from build123d import *

# Parameters (mm, degrees)
SKETCH1_R                     = 22.5
PLATE_DEPTH                   = 5
OPENING_START                 = 1.5
OPENING_FOR_SCREW_DEPTH       = 5
SKETCH7_R                     = 1.75
SCREW_HOLE_DEPTH              = 5
CIRPATTERN20_COUNT            = 3
SKETCH10_W                    = 45
SKETCH10_H                    = 1
SKETCH10_W_2                  = 1
SKETCH10_H_2                  = 45
CUT_EXTRUDE5_DEPTH            = 1
CUT_EXTRUDE6_DEPTH            = 1
SKETCH12_W                    = 10
SKETCH12_H                    = 10
SKETCH12_W_2                  = 5
SKETCH12_H_2                  = 5
TOOL_CONNECT_PIECE_DEPTH      = 10
TOOL_CONNECT_PIECE_DEPTH_BACK = 1
SKETCH14_R                    = 1.5
CUT_EXTRUDE8_DEPTH            = 10
SKETCH15_R                    = 1.5
CUT_EXTRUDE9_DEPTH            = 28.5


with BuildPart() as part:
    # Sketch1 → plate (new body)
    with BuildSketch(Plane(origin=(0, 0, 0), x_dir=(1, 0, 0), z_dir=(0, 1, 0))):
        Circle(SKETCH1_R)
    extrude(amount=PLATE_DEPTH)

    # Sketch6 → opening for screw (cut)
    with BuildSketch(Plane(origin=(0, 5, 0), x_dir=(1, 0, 0), z_dir=(0, 1, 0)).offset(OPENING_START)):
        with BuildLine():
            Line((-4, -22.5), (-4, -18.4))
            ThreePointArc((-4, -18.4), (0, -14.4), (4, -18.4))
            Line((4, -18.4), (4, -22.5))
            ThreePointArc((4, -22.5), (0, -26.5), (-4, -22.5))
        make_face()
    opening_for_screw = extrude(amount=-OPENING_FOR_SCREW_DEPTH, mode=Mode.SUBTRACT)

    # Sketch7 → screw hole (cut)
    with BuildSketch(Plane(origin=(0, 1.5, 0), x_dir=(1, 0, 0), z_dir=(0, 1, 0))):
        with Locations((0, -18.4)):
            Circle(SKETCH7_R)
    screw_hole = extrude(amount=-SCREW_HOLE_DEPTH, mode=Mode.SUBTRACT)

    # CirPattern20: opening for screw, screw hole ×3 about axis
    cirpattern20_axis = Axis((0, 0, 0), (0, 1, 0))
    for i in range(1, CIRPATTERN20_COUNT):
        add(opening_for_screw.rotate(cirpattern20_axis, i * 360 / CIRPATTERN20_COUNT), mode=Mode.SUBTRACT)
        add(screw_hole.rotate(cirpattern20_axis, i * 360 / CIRPATTERN20_COUNT), mode=Mode.SUBTRACT)

    # Sketch10 → Cut-Extrude5 (cut)
    with BuildSketch(Plane(origin=(0, 5, 0), x_dir=(1, 0, 0), z_dir=(0, 1, 0))):
        Rectangle(SKETCH10_W, SKETCH10_H)
        Rectangle(SKETCH10_W_2, SKETCH10_H_2)
    extrude(amount=-CUT_EXTRUDE5_DEPTH, mode=Mode.SUBTRACT)

    # Sketch11 → Cut-Extrude6 (cut)
    with BuildSketch(Plane(origin=(0, 5, 0), x_dir=(1, 0, 0), z_dir=(0, 1, 0))):
        Polygon((2.616666667, 13.742425761), (2.616666667, 15.289220632), (3.675, 15.289220632), (3.675, 13.742425761), (5.303205128, 13.742425761), (5.303205128, 12.684092427), (3.675, 12.684092427), (3.675, 11.137297556), (2.616666667, 11.137297556), (2.616666667, 12.684092427), (0.988461538, 12.684092427), (0.988461538, 13.742425761), align=None)
        Polygon((6.136388221, 16.510374479), (7.479657452, 16.510374479), (8.806390224, 14.471301963), (10.135667067, 16.510374479), (11.480208333, 16.510374479), (9.47802484, 13.43968137), (11.6125, 10.160374479), (10.269230769, 10.160374479), (8.806390224, 12.409332812), (7.339733574, 10.160374479), (5.995192308, 10.160374479), (8.134755609, 13.440953405), align=None)
        Polygon((-18.458103671, -3.794817635), (-18.458103671, -2.248022763), (-17.399770338, -2.248022763), (-17.399770338, -3.794817635), (-15.771565209, -3.794817635), (-15.771565209, -4.853150968), (-17.399770338, -4.853150968), (-17.399770338, -6.39994584), (-18.458103671, -6.39994584), (-18.458103671, -4.853150968), (-20.086308799, -4.853150968), (-20.086308799, -3.794817635), align=None)
        Polygon((-15.07957803, -1.026868917), (-13.811358879, -1.026868917), (-12.677975466, -3.254202651), (-11.544592052, -1.026868917), (-10.276372902, -1.026868917), (-12.108103671, -4.626728693), (-12.108103671, -7.376868917), (-13.247847261, -7.376868917), (-13.247847261, -4.626728693), align=None)
    extrude(amount=-CUT_EXTRUDE6_DEPTH, mode=Mode.SUBTRACT)

    # Sketch12 → tool connect piece (add, two sides)
    with BuildSketch(Plane(origin=(0, 5, 0), x_dir=(1, 0, 0), z_dir=(0, 1, 0))) as tool_connect_piece_sk:
        Rectangle(SKETCH12_W, SKETCH12_H)
        Rectangle(SKETCH12_W_2, SKETCH12_H_2, mode=Mode.SUBTRACT)
    extrude(amount=TOOL_CONNECT_PIECE_DEPTH)
    extrude(tool_connect_piece_sk.sketch, amount=-TOOL_CONNECT_PIECE_DEPTH_BACK)

    # Sketch14 → Cut-Extrude8 (cut)
    with BuildSketch(Plane(origin=(0, 0, -5), x_dir=(-1, 0, 0), z_dir=(0, 0, -1))):
        with Locations((0, 10)):
            Circle(SKETCH14_R)
    extrude(amount=-CUT_EXTRUDE8_DEPTH, mode=Mode.SUBTRACT)

    # Sketch15 → Cut-Extrude9 (cut, through all)
    with BuildSketch(Plane(origin=(5, 0, 0), x_dir=(0, 0, -1), z_dir=(1, 0, 0))):
        with Locations((0, 10)):
            Circle(SKETCH15_R)
    extrude(amount=-CUT_EXTRUDE9_DEPTH, mode=Mode.SUBTRACT)


solid = part.part
Could you check a few things on this model? Use its own coordinates, in mm. A direction names the side the tool comes from. Give positions to 0.01 mm unless a question says otherwise; leave off trailing zeros. Order: outer loops, then holes, each group sorted by start corner. A loop starts at its lowest first (then second) coordinate and runs counter-clockwise, first axis right, second up.
1. I need wall thicknesses on L1, parallel to Z at x = 0, y = 1.1; L2, parallel to X at y = 5.25, z = 1.5; L3, parallel to Y at x = -3, z = 0. Which ranges of each line are inside material? Lowest first, please.
Answers below:
L1: z = -22.5 to 16.65, 20.15 to 22.5
L2: x = -5 to -2.5, 2.5 to 5
L3: y = 0 to 8.5, 11.5 to 15
2. Thinking about a two-plate mould opening in X: for faces 4 (the flat face through (14, 4, 0)), 5 (the flat face through (3.2, 4.5, -11.137)), 6 (the flat face through (15.532, 3.274, -13.586)), 7 (the flat face through (-0.5, 4.5, 1.5)), which applies, +X half, -X half, draft (parallel to the pull), parting line (faces both ways), or undercut?
Answers below:
face 4: draft
face 5: undercut
face 6: +X half
face 7: undercut
3. Suppose I cut it at D-D (x = 12.5). Write out the boundary of the cut face in (y, z).
Answers below:
outline: (0, -18.71) - (5, -18.71) - (5, -11.25) - (1.5, -11.25) - (1.5, -7.15) - (5, -7.15) - (5, -0.5) - (4, -0.5) - (4, 0.5) - (5, 0.5) - (5, 18.71) - (0, 18.71) - close
4. Suppose I cut it at C-C (z = -19). Write out the boundary of the cut face in (x, y).
Answers below:
outline: (-12.05, 0) - (12.05, 0) - (12.05, 5) - (0.5, 5) - (0.5, 4) - (-0.5, 4) - (-0.5, 5) - (-12.05, 5) - close
5. Suppose I cut it at B-B (y = 6.75). Write out the boundary of the cut face in (x, z).
Answers below:
outline: (-5, -5) - (5, -5) - (5, 5) - (-5, 5) - close; hole (-2.5, -2.5) - (2.5, -2.5) - (2.5, 2.5) - (-2.5, 2.5) - close
6. Which directions (+Z, -Z, +X, -X, +Y, -Y) give clear straight access to the entire face, cutting with the end or side of a thin tool? Please do faces 1 (the flat face through (0.5, 4.5, -13.6)), 2 (the flat face through (-0.8, 1.5, 20.2)), 3 (the flat face through (9, 4, -13)).
Answers below:
face 1: -Z, +Y
face 2: +Z, +Y
face 3: +Y
7. For pin 1 (0.8 mm diameter, centred on y = 4.5, z = -1, fed in from +X); pin 2 (1.1 mm diameter, centred on y = 4.5, z = -13.5, fed in from +X); pin 3 (6 mm diameter, centred on y = 7.5, z = -14.5, fed in from +X), each with a flat end and sliding along its axis, tell me the tip position at first contact or that it passes through.
Answers below:
pin 1: stops at x = 22.49
pin 2: stops at x = 16.34
pin 3: stops at x = 17.18
8. Suppose I cut it at A-A (y = 10). Write out the boundary of the cut face in (x, z).
Answers below:
outline: (-5, -5) - (-1.5, -5) - (-1.5, -2.5) - (-2.5, -2.5) - (-2.5, -1.5) - (-5, -1.5) - close; (-5, 1.5) - (-2.5, 1.5) - (-2.5, 2.5) - (-1.5, 2.5) - (-1.5, 5) - (-5, 5) - close; (1.5, -5) - (5, -5) - (5, -1.5) - (2.5, -1.5) - (2.5, -2.5) - (1.5, -2.5) - close; (1.5, 2.5) - (2.5, 2.5) - (2.5, 1.5) - (5, 1.5) - (5, 5) - (1.5, 5) - close
